from build123d import *

# Parameters (mm, degrees)
F0_R         = 10.3
F1_DEPTH     = 9
F3_R         = 3.1
F4_DEPTH     = 9.001
F6_DEPTH     = 1.8
F7_T4_ANGLE  = 359.64
F7_S5_R      = 3.1
F7_T6_DEPTH  = 5
F7_T10_ANGLE = 359.64
F7_S11_R     = 3.1
F7_T12_DEPTH = 5
F7_T16_ANGLE = 359.64
F7_S17_R     = 3.1
F7_T18_DEPTH = 5
F9_R         = 12.75
F10_DEPTH    = 25
F11_R        = 3.1
F12_DEPTH    = 34.0010001
F13_R        = 12.75
F13_R_2      = 11.35
F14_DEPTH    = 20
F16_DEPTH    = 5
F17_R        = 10.3
F18_DEPTH    = 34.0010001
F20_START    = -5
F20_DEPTH    = 5


# Not quite as in the source:
# - a fillet or chamfer that OpenCascade refuses, or shapes differently, is made with other operations: its cross-section is extruded or revolved along the edge and cut away or added


with BuildPart() as f1:
    # F0 (on Front) → F1 (new body)
    with BuildSketch(Plane.XZ):
        Circle(F0_R)
    extrude(amount=F1_DEPTH)

    # F3 (on face) → F4 (cut, through all)
    with BuildSketch(Plane.XZ.offset(9)):
        Circle(F3_R)
    extrude(amount=-F4_DEPTH, mode=Mode.SUBTRACT)

    # F5 (on face) → F6 (cut)
    with BuildSketch(Plane.XZ.offset(9)):
        with BuildLine():
            ThreePointArc((-3.0819681678, 0.333874546), (-2.6846787517, 1.55), (-1.8301279224, 2.502125454))
            ThreePointArc((-1.8301279224, 2.502125454), (-6.4951905284, 3.75), (-3.0819681678, 0.333874546))
        make_face()
        with BuildLine():
            ThreePointArc((6.8301270189, 2.5), (4.331189746, 4.9999997741), (1.8301279224, 2.502125454))
            ThreePointArc((1.8301279224, 2.502125454), (2.6846787517, 1.55), (3.0819681678, 0.333874546))
            ThreePointArc((3.0819681678, 0.333874546), (5.5810472546, 0.3354680497), (6.8301270189, 2.5))
        make_face()
        with BuildLine():
            ThreePointArc((1.2518402454, -2.836), (0, -3.1), (-1.2518402454, -2.836))
            ThreePointArc((-1.2518402454, -2.836), (-1.2490795384, -7.1655946774), (2.5, -5))
            ThreePointArc((2.5, -5), (2.1655946774, -3.7509204616), (1.2518402454, -2.836))
        make_face()
    extrude(amount=-F6_DEPTH, mode=Mode.SUBTRACT)

    # F7: fillet of radius 1 on 3 edges, made by hand


with BuildPart() as f7_tool2:
    # F7_s3 → F7_t4 (revolve)
    with BuildSketch(Plane(origin=(0.0078111935, 0, 0.0136280797), x_dir=(0, 1, 0), z_dir=(-0.497276838, 0, -0.8675919239))):
        with BuildLine():
            ThreePointArc((-8.2, -2.499975326), (-7.4928932188, -2.7928685448), (-7.2, -3.499975326))
            Line((-7.2, -3.499975326), (-7.18, -3.499975326))
            Line((-7.18, -3.499975326), (-7.18, -2.479975326))
            Line((-7.18, -2.479975326), (-8.2, -2.479975326))
            Line((-8.2, -2.479975326), (-8.2, -2.499975326))
        make_face()
    revolve(axis=Axis((-4.3301270189, -7.2, 2.5), (0, -1, 0)), revolution_arc=F7_T4_ANGLE)

    # F7_s5 → F7_t6 (cut, symmetric)
    with BuildSketch(Plane.XZ.offset(7.7)):
        Circle(F7_S5_R)
    extrude(amount=F7_T6_DEPTH, both=True, mode=Mode.SUBTRACT)


with BuildPart() as f1_1:
    add(f1.part)

    # F7_t1: union F7_tool2
    add(f7_tool2.part)


with BuildPart() as f7_tool8:
    # F7_s9 → F7_t10 (revolve)
    with BuildSketch(Plane(origin=(0.0078966665, 0, -0.0135787318), x_dir=(0, 1, 0), z_dir=(-0.5027182272, 0, 0.8644503364))):
        with BuildLine():
            ThreePointArc((-8.2, -2.499975326), (-7.4928932188, -2.7928685448), (-7.2, -3.499975326))
            Line((-7.2, -3.499975326), (-7.18, -3.499975326))
            Line((-7.18, -3.499975326), (-7.18, -2.479975326))
            Line((-7.18, -2.479975326), (-8.2, -2.479975326))
            Line((-8.2, -2.479975326), (-8.2, -2.499975326))
        make_face()
    revolve(axis=Axis((4.3301270189, -7.2, 2.5), (0, -1, 0)), revolution_arc=F7_T10_ANGLE)

    # F7_s11 → F7_t12 (cut, symmetric)
    with BuildSketch(Plane.XZ.offset(7.7)):
        Circle(F7_S11_R)
    extrude(amount=F7_T12_DEPTH, both=True, mode=Mode.SUBTRACT)


with BuildPart() as f1_2:
    add(f1_1.part)

    # F7_t7: union F7_tool8
    add(f7_tool8.part)


with BuildPart() as f7_tool14:
    # F7_s15 → F7_t16 (revolve)
    with BuildSketch(Plane(origin=(-0.0157078599, 0, -4.93479e-05), x_dir=(0, 1, 0), z_dir=(0.9999950652, 0, 0.0031415875))):
        with BuildLine():
            ThreePointArc((-8.2, -2.499975326), (-7.4928932188, -2.7928685448), (-7.2, -3.499975326))
            Line((-7.2, -3.499975326), (-7.18, -3.499975326))
            Line((-7.18, -3.499975326), (-7.18, -2.479975326))
            Line((-7.18, -2.479975326), (-8.2, -2.479975326))
            Line((-8.2, -2.479975326), (-8.2, -2.499975326))
        make_face()
    revolve(axis=Axis((0, -7.2, -5), (0, -1, 0)), revolution_arc=F7_T16_ANGLE)

    # F7_s17 → F7_t18 (cut, symmetric)
    with BuildSketch(Plane.XZ.offset(7.7)):
        Circle(F7_S17_R)
    extrude(amount=F7_T18_DEPTH, both=True, mode=Mode.SUBTRACT)


with BuildPart() as f1_3:
    add(f1_2.part)

    # F7_t13: union F7_tool14
    add(f7_tool14.part)

    # F9 (on offset) → F10 (join)
    with BuildSketch(Plane(origin=(0, 0, 0), x_dir=(-1, 0, 0), z_dir=(0, 1, 0))):
        Circle(F9_R)
    extrude(amount=F10_DEPTH)

    # F11 (on face) → F12 (cut, through all)
    with BuildSketch(Plane(origin=(0, 25, 0), x_dir=(-1, 0, 0), z_dir=(0, 1, 0))):
        Circle(F11_R)
    extrude(amount=-F12_DEPTH, mode=Mode.SUBTRACT)

    # F13 (on face) → F14 (cut)
    with BuildSketch(Plane(origin=(0, 25, 0), x_dir=(-1, 0, 0), z_dir=(0, 1, 0))):
        Circle(F13_R)
        Circle(F13_R_2, mode=Mode.SUBTRACT)
    extrude(amount=-F14_DEPTH, mode=Mode.SUBTRACT)

    # F15 (on face) → F16 (join)
    with BuildSketch(Plane(origin=(0, 5, 0), x_dir=(-1, 0, 0), z_dir=(0, 1, 0))):
        with BuildLine():
            ThreePointArc((2, 12.5921602595), (0, 12.75), (-2, 12.5921602595))
            Line((-2, 12.5921602595), (-2, 11.1723990262))
            ThreePointArc((-2, 11.1723990262), (0, 11.35), (2, 11.1723990262))
            Line((2, 11.1723990262), (2, 12.5921602595))
        make_face()
        with BuildLine():
            ThreePointArc((2, -11.1723990262), (0, -11.35), (-2, -11.1723990262))
            Line((-2, -11.1723990262), (-2, -12.5921602595))
            ThreePointArc((-2, -12.5921602595), (0, -12.75), (2, -12.5921602595))
            Line((2, -12.5921602595), (2, -11.1723990262))
        make_face()
    extrude(amount=F16_DEPTH)

    # F17 (on face) → F18 (cut, through all)
    with BuildSketch(Plane.XZ.offset(9)):
        Circle(F17_R)
    extrude(amount=-F18_DEPTH, mode=Mode.SUBTRACT)

    # F19 (on face) → F20 (join)
    with BuildSketch(Plane(origin=(0, 25, 0), x_dir=(-1, 0, 0), z_dir=(0, 1, 0)).offset(F20_START)):
        with BuildLine():
            Line((-7.5, 0), (-10.3, 0))
            ThreePointArc((-10.3, 0), (-9.5744451536, -3.7973675092), (-7.5, -7.0597450379))
            Line((-7.5, -7.0597450379), (-7.5, 0))
        make_face()
    extrude(amount=-F20_DEPTH)


solid = f1_3.part
Model file for the job. Use its own axes, mm. A direction names the side the tool comes from. Give positions to 0.01 mm unless a question says otherwise; leave off trailing zeros. Loops run counter-clockwise (first coordinate to the right, second up) from the corner with the lowest first, then second, coordinate; pieces in that order, holes last.
1) Saw through at B-B (z = 6.5). Write the cut outline in (x, y), plus the area to 3 significant figures.
2) Flat gauge pins, fed straight in: pin 1 Ø3 at (x, z) = (-0.5, -9.5) entering from +Y; pin 2 Ø6 at (x, z) = (4, 0.5) entering from -Y; pin 3 Ø1.5 at (y, z) = (5, -4.5) entering from -X; pin 4 Ø1.4 at (x, z) = (9, -2.5) entering from -Y. Where does each tip first touch, or does it go through?
3) Wall check: line 1 (Z direction, x = 0, y = 14.5); line 2 (Z direction, x = 0, y = 8.75). Give the ranges that are in metal, low to high.
4) Saw through at C-C (y = 23). Write the cut outline in (x, z).
5) Tool access for faces 4 (the flat face through (2, 7, -12)), 5 (the flat face through (-2, 7, 12)), 6 (the cylindrical face through (-5.24, 15.14, -10.07)), 7 (the flat face through (9, 18, 0)), 8 (the flat face through (-2, 7, -12)): list every direction of +Z, -Z, +X, -X, +Y, -Y with a clear straight run to the whole face (end or side of a thin tool).
6) Saw through at A-A (x = 0). Write the cut outline in (y, z).
7) Pull direction X, two halves, no side cores. Call faces 1 (the flat face through (7.5, 18, -4)), 2 (the flat face through (2, 7, 12)), 3 (the flat face through (0, 10, -12)): +X half, -X half, draft (parallel to the pull), parting line (faces both ways), or undercut.
Answer block:
1. outline: (-10.97, 0) - (-7.99, 0) - (-7.99, 25) - (-9.3, 25) - (-9.3, 5) - (-10.97, 5) - close; (7.99, 0) - (10.97, 0) - (10.97, 5) - (9.3, 5) - (9.3, 25) - (7.99, 25) - close
1. area: 82.4 mm2
2. pin 1: stops at y = 25
2. pin 2: passes through
2. pin 3: stops at x = -12.19
2. pin 4: stops at y = 15
3. line 1: z = -11.35 to -10.3, 10.3 to 11.35
3. line 2: z = -12.75 to -10.3, 10.3 to 12.75
4. outline: circle Ø22.7 at (0, 0); hole circle Ø20.6 at (0, 0)
5. face 4: -Z, +X, +Y
5. face 5: +Z, -X, +Y
5. face 6: +Y
5. face 7: +Y, -Y
5. face 8: -Z, -X, +Y
6. outline: (0, -12.75) - (10, -12.75) - (10, -11.35) - (25, -11.35) - (25, -10.3) - (0, -10.3) - close; (0, 10.3) - (25, 10.3) - (25, 11.35) - (10, 11.35) - (10, 12.75) - (0, 12.75) - close
7. face 1: undercut
7. face 2: +X half
7. face 3: draft
